Design review of the part built by this model. Coordinates are the model's own, in mm. A direction names the side the tool comes from. Round coordinates to 2 decimals unless told otherwise and drop trailing zeros. Order: outer loops, then holes, each group sorted by start corner. A loop starts at its lowest first (then second) coordinate and runs counter-clockwise, first axis right, second up. Notation, with made-up numbers: (39, -9) - (75, -9) arc R22 ccw to (75, 6) - close; hole circle Ø11 at (87.25, 7). An arc over 180 degrees is marked (long way). Use CSV: the item, a comma, the result in double quotes.
from build123d import *


with BuildPart() as part:
    # Esquisse1 → Révolution1 (revolve)
    with BuildSketch(Plane.XY, mode=Mode.PRIVATE) as r_volution1_sk:
        with BuildLine():
            Line((1.25, 13.5), (1.25, 0.5))
            ThreePointArc((1.25, 0.5), (0.673145601, 0.129635998), (0, 0))
            Line((0, 0), (0, 14.5))
            Line((0, 14.5), (1.401923789, 14.5))
            ThreePointArc((1.401923789, 14.5), (2.901923789, 14.098076211), (4, 13))
            Line((4, 13), (3, 13))
            Line((3, 13), (3, 13.5))
            Line((3, 13.5), (1.25, 13.5))
        make_face()
    revolve(r_volution1_sk.sketch.rotate(Axis((0, 0, 0), (0, 1, 0)), 90), axis=Axis((0, 0, 0), (0, 1, 0)))


solid = part.part
1) Insertion check: pin 1 Ø1.5 at (x, y) = (-1.5, 4) entering from -Z; pin 2 Ø4 at (x, y) = (-2.5, 4.5) entering from -Z; pin 3 Ø2 at (y, z) = (2, 0.5) entering from -X; pin 4 Ø1.5 at (x, y) = (-3, 9.5) entering from +Z. Each pin has a flat end and moves straight along its axis. Give the tip position at first contact, or say it passes through.
Data:
pin 1,"stops at z = -1"
pin 2,"stops at z = -1.15"
pin 3,"stops at x = -1.25"
pin 4,"passes through"
2) We need section A-A (y = 11). Give the boundary of the cut face in (x, z).
Data:
outline,"circle Ø2.5 at (0, 0)"
3) To check wall thickness, follow L1, parallel to X at y = 13.3, z = 0; L2, parallel to X at y = 13.4, z = 0; L3, parallel to Y at x = 3.25, z = 0.5. State the ranges of each line that lie inside material, in increasing order. Write a range as from..to.
Data:
L1,"x = -3.8..-3, -1.25..1.25, 3..3.8"
L2,"x = -3.72..-3, -1.25..1.25, 3..3.72"
L3,"y = 13..13.83"
4) The part is to be moulded in two halves that separate along Z. For faces 3 (the face through (-0.9, 13.25, -2.86)), 4 (the face through (1, 13.5, -1)), 5 (the face through (-3, 13, -1)), say which applies: +Z half, -Z half, draft (parallel to the pull), parting line (faces both ways), or undercut.
Data:
face 3,"undercut"
face 4,"undercut"
face 5,"draft"
5) For faces 1 (the face through (0, 14.5, 0)), 2 (the face through (-0.05, 6.91, 1.25)), list the 3-axis set-ups (+Z, -Z, +X, -X, +Y, -Y) from which the entire face can be reached by the end or side of a thin tool; tool diameter is ignored.
Data:
face 1,"+Z, -Z, +X, -X, +Y"
face 2,"-Y"
